Source: CAD feature listing. Evaluate the final solid. Frame: model axes, mm. A direction names the side the tool comes from. Round coordinates to 2 decimals unless told otherwise and drop trailing zeros. Loops run counter-clockwise (first coordinate to the right, second up) from the corner with the lowest first, then second, coordinate; pieces in that order, holes last.
(1) Section A-A, the plane z = -11. Return the cut outline in (x, y).
(2) Section B-B, the plane y = 0. Return the cut outline in (x, z).
(3) Mould query, pull axis Y, two halves, no side actions, for faces 4 (the flat face through (-32, 25, -16)), 5 (the flat face through (40, 0, 2)), 6 (the flat face through (3, -25, 2)). Classes: pulls with the +Y half, pulls with the -Y half, needs draft (parallel to the pull), parting line crosses it, or undercut.
(4) Section C-C, the plane x = 11.5. Return the cut outline in (y, z).
(5) Set-up query: faces 1 (the cylindrical face through (-22.9, -17.4, 1.5)), 2 (the flat face through (-9, 0, 3.5)), 3 (the flat face through (-32, -25, -16)). Return all of +Z, -Z, +X, -X, +Y, -Y with unobstructed straight access to the full face (end or side cutting, diameter ignored); none if empty.
(6) Section D-D, the plane z = -23.5. Return the cut outline in (x, y).
(7) First-contact query: pin 1 Ø4 at (x, y) = (22, 12) entering from -Z; pin 2 Ø5 at (x, y) = (-27.5, 3) entering from -Z; pin 3 Ø4 at (x, y) = (-22, 5) entering from -Z; pin 4 Ø1.8 at (y, z) = (-26, -7) entering from +X. Flat tips, straight axial feed; report the tip coordinate or a pass-through.
(8) Material intervals for probe 1 along Y at (x, z) = (15, 2); probe 2 along Y at (x, z) = (-35, -1.5); probe 3 along Z at (x, y) = (-34, 4.5), sorted ascending.
```python
from build123d import *

# Parameters (mm, degrees)
SKETCH_1_W          = 80
SKETCH_1_H          = 50
EXTRUDE_1_DEPTH     = 3.5
CUT_EXTRUDE_1_DEPTH = 3
SKETCH_12_W         = 17.020417597
SKETCH_12_H         = 35
EXTRUDE_2_DEPTH     = 3.5
FILLET_1_R          = 1
FILLET_2_R          = 5
SKETCH_13_R         = 3
CUT_EXTRUDE_2_DEPTH = 10
SKETCH_14_R         = 17
CUT_EXTRUDE_3_DEPTH = 8
FILLET_3_R          = 10


with BuildPart() as part:
    # 草图1 → 凸台-拉伸1 (new body)
    with BuildSketch(Plane.XY):
        Rectangle(SKETCH_1_W, SKETCH_1_H)
    extrude(amount=EXTRUDE_1_DEPTH)

    # 草图2 → 切除-拉伸1 (cut)
    with BuildSketch(Plane(origin=(0, 0, 0), x_dir=(-1, 0, 0), z_dir=(0, 0, -1))):
        with BuildLine():
            Line((27.979582403, -12.4), (27.983580804, 12.6))
            ThreePointArc((27.983580804, 12.6), (22.879562421, 17.602998701), (17.979582403, 12.4))
            Line((17.979582403, 12.4), (17.979582403, -12.4))
            ThreePointArc((17.979582403, -12.4), (22.979582403, -17.4), (27.979582403, -12.4))
        make_face()
    extrude(amount=-CUT_EXTRUDE_1_DEPTH, mode=Mode.SUBTRACT)

    # 草图12 → 凸台-拉伸2 (add)
    with BuildSketch(Plane(origin=(0, 25, 0), x_dir=(1, 0, 0), z_dir=(0, 1, 0))):
        with Locations((-31.489791202, 14)):
            Rectangle(SKETCH_12_W, SKETCH_12_H)
    extrude_2 = extrude(amount=EXTRUDE_2_DEPTH)

    # 镜向1: 凸台-拉伸2 across plane
    add(extrude_2.mirror(Plane.ZX))

    # 圆角1
    fillet_1_edges = [part.edges().sort_by_distance(p)[0] for p in [
        (-31.489791201, 28.5, 3.5),
        (-31.489791201, -28.5, 3.5),
    ]]
    fillet(fillet_1_edges, radius=FILLET_1_R)

    # 圆角2
    fillet_2_edges = [part.edges().sort_by_distance(p)[0] for p in [
        (-22.979582403, -26.75, -31.5),
        (-40, -26.75, -31.5),
        (-40, 26.75, -31.5),
        (-22.979582403, 26.75, -31.5),
    ]]
    fillet(fillet_2_edges, radius=FILLET_2_R)

    # 草图13 → 切除-拉伸2 (cut)
    with BuildSketch(Plane(origin=(0, 28.5, 0), x_dir=(1, 0, 0), z_dir=(0, 1, 0))):
        with Locations(Location((-31.229582403, 23.5, 0), (0, 0, 270))):
            Circle(SKETCH_13_R)
    cut_extrude_2 = extrude(amount=-CUT_EXTRUDE_2_DEPTH, mode=Mode.SUBTRACT)

    # 镜向2: 切除-拉伸2 across plane
    add(cut_extrude_2.mirror(Plane.ZX), mode=Mode.SUBTRACT)

    # 草图14 → 切除-拉伸3 (cut)
    with BuildSketch(Plane(origin=(0, 0, 0), x_dir=(-1, 0, 0), z_dir=(0, 0, -1))):
        with Locations((-15, 0)):
            Circle(SKETCH_14_R)
    extrude(amount=-CUT_EXTRUDE_3_DEPTH, mode=Mode.SUBTRACT)

    # 圆角3
    fillet_3_edges = [part.edges().sort_by_distance(p)[0] for p in [
        (40, -25, 1.75),
        (40, 25, 1.75),
    ]]
    fillet(fillet_3_edges, radius=FILLET_3_R)


solid = part.part
```
Output values:
1. outline: (-40, -28.5) - (-22.98, -28.5) - (-22.98, -25) - (-40, -25) - close; (-40, 25) - (-22.98, 25) - (-22.98, 28.5) - (-40, 28.5) - close
2. outline: (-40, 0) - (-27.98, 0) - (-27.98, 3) - (-17.98, 3) - (-17.98, 0) - (-2, 0) - (-2, 3.5) - (-40, 3.5) - close; (32, 0) - (40, 0) - (40, 3.5) - (32, 3.5) - close
3. face 4: undercut
3. face 5: needs draft
3. face 6: pulls with the -Y half
4. outline: (-25, 0) - (-16.64, 0) - (-16.64, 3.5) - (-25, 3.5) - close; (16.64, 0) - (25, 0) - (25, 3.5) - (16.64, 3.5) - close
5. face 1: -Z
5. face 2: +Z, +X, -X, +Y, -Y
5. face 3: -Z, +X, -X
6. outline: (-40, -28.5) - (-34.23, -28.5) - (-34.23, -25) - (-40, -25) - close; (-40, 25) - (-34.23, 25) - (-34.23, 28.5) - (-40, 28.5) - close; (-28.23, -28.5) - (-22.98, -28.5) - (-22.98, -25) - (-28.23, -25) - close; (-28.23, 25) - (-22.98, 25) - (-22.98, 28.5) - (-28.23, 28.5) - close
7. pin 1: passes through
7. pin 2: stops at z = 0
7. pin 3: stops at z = 3
7. pin 4: stops at x = -22.98
8. probe 1: y = -25 to -17, 17 to 25
8. probe 2: y = -28.5 to -25, 25 to 28.5
8. probe 3: z = 0 to 3.5
